For this review, take the finished solid that the model builds, in its own axes (mm). Face numbers are marked on the shaded views. A direction names the side the tool comes from. Coordinates: 2 decimals unless noted, no trailing zeros. Order: outer loops, then holes, each group sorted by start corner. A loop starts at its lowest first (then second) coordinate and runs counter-clockwise, first axis right, second up. Notation, with made-up numbers: M 46.5,20 L 78.5,20 A19 cw 78.5,38 Z; hole C 48.25,38.25 d6. An arc over 180 degrees is marked long. Use CSV: the item, a comma, the result in double quotes.
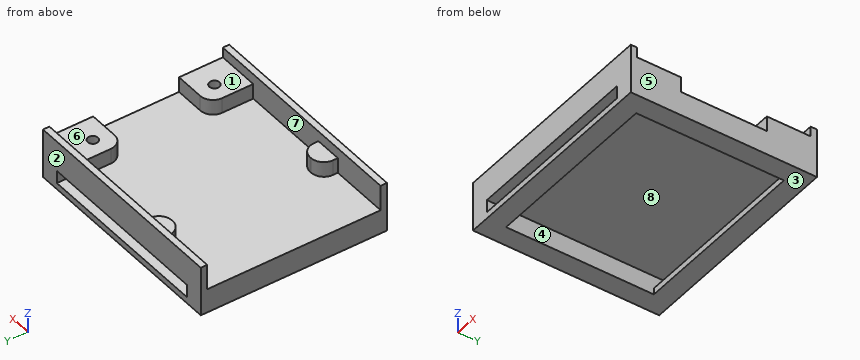
```python
from build123d import *

# Parameters (mm, degrees)
SKETCH2_W               = 29.17
SKETCH2_H               = 34.29
BOSS_EXTRUDE1_DEPTH     = 0.8
SKETCH4_W               = 4.2
SKETCH4_H               = 2.75
SKETCH4_W_2             = 6.61
SKETCH4_H_2             = 6.86
BOSS_EXTRUDE3_DEPTH     = 2.4
SKETCH5_W               = 34.29
SKETCH5_H               = 1
BOSS_EXTRUDE5_DEPTH     = 4
SKETCH6_W               = 3.01
SKETCH6_H               = 29.17
BOSS_EXTRUDE6_DEPTH     = 2
CUT_EXTRUDE1_DEPTH      = 24.10223474
CUT_EXTRUDE1_DEPTH_BACK = 24.10223474
SKETCH8_R               = 0.8
SKETCH9_W               = 34.29
SKETCH9_H               = 29.17
SKETCH9_W_2             = 28.27
SKETCH9_H_2             = 23.15
BOSS_EXTRUDE8_DEPTH     = 1
FILLET1_R               = 2


with BuildPart() as part:
    # Sketch2 → Boss-Extrude1 (new body)
    with BuildSketch(Plane(origin=(0, 0, 0), x_dir=(0, 1, 0), z_dir=(0, 0, 1))):
        Rectangle(SKETCH2_W, SKETCH2_H)
    extrude(amount=BOSS_EXTRUDE1_DEPTH)

    # Sketch4 → Boss-Extrude3 (add)
    with BuildSketch(Plane.XY.offset(0.8)):
        with Locations((-5.745, -12.21)):
            Rectangle(SKETCH4_W, SKETCH4_H)
        with Locations((13.84, -10.155)):
            Rectangle(SKETCH4_W_2, SKETCH4_H_2)
        with Locations((13.84, 10.155)):
            Rectangle(SKETCH4_W_2, SKETCH4_H_2)
        with Locations((-5.745, 12.21)):
            Rectangle(SKETCH4_W, SKETCH4_H)
    extrude(amount=BOSS_EXTRUDE3_DEPTH)

    # Sketch5 → Boss-Extrude5 (add)
    with BuildSketch(Plane.XY.offset(0.8)):
        with Locations((0, 14.085)):
            Rectangle(SKETCH5_W, SKETCH5_H)
        with Locations((0, -14.085)):
            Rectangle(SKETCH5_W, SKETCH5_H)
    extrude(amount=BOSS_EXTRUDE5_DEPTH)

    # Sketch6 → Boss-Extrude6 (add)
    with BuildSketch(Plane(origin=(0, 0, 0), x_dir=(1, 0, 0), z_dir=(0, 0, -1))):
        with Locations((15.64, 0)):
            Rectangle(SKETCH6_W, SKETCH6_H)
        with Locations((-15.64, 0)):
            Rectangle(SKETCH6_W, SKETCH6_H)
    extrude(amount=BOSS_EXTRUDE6_DEPTH)

    # Sketch8 → Cut-Extrude1 (cut, two sides: drawn at the far end of the back side and taken through both)
    with BuildSketch(Plane.XY.offset(3.2).offset(-CUT_EXTRUDE1_DEPTH_BACK)):
        with Locations((13.335, 9.525)):
            Circle(SKETCH8_R)
        with Locations((13.335, -9.525)):
            Circle(SKETCH8_R)
    extrude(amount=CUT_EXTRUDE1_DEPTH + CUT_EXTRUDE1_DEPTH_BACK, mode=Mode.SUBTRACT)

    # Sketch9 → Boss-Extrude8 (add)
    with BuildSketch(Plane(origin=(0, 0, -2), x_dir=(1, 0, 0), z_dir=(0, 0, -1))):
        Rectangle(SKETCH9_W, SKETCH9_H)
        Rectangle(SKETCH9_W_2, SKETCH9_H_2, mode=Mode.SUBTRACT)
    extrude(amount=BOSS_EXTRUDE8_DEPTH)

    # Fillet1
    fillet1_edges = [part.edges().sort_by_distance(p)[0] for p in [
        (-7.845, 10.835, 2),
        (-3.645, 10.835, 2),
        (10.535, 6.725, 2),
        (10.535, -6.725, 2),
        (-3.645, -10.835, 2),
        (-7.845, -10.835, 2),
    ]]
    fillet(fillet1_edges, radius=FILLET1_R)


solid = part.part
```
Item 1: Add section B-B on z = 1.5. State the section outline as (x, y) points (3 decimals).
Solutions:
outline,"M -17.145,-14.585 L 17.145,-14.585 L 17.145,-6.725 L 12.535,-6.725 A2 ccw 10.535,-8.725 L 10.535,-13.585 L -3.645,-13.585 L -3.645,-12.835 A2 ccw -5.645,-10.835 L -5.845,-10.835 A2 ccw -7.845,-12.835 L -7.845,-13.585 L -17.145,-13.585 Z; M -17.145,13.585 L -7.845,13.585 L -7.845,12.835 A2 ccw -5.845,10.835 L -5.645,10.835 A2 ccw -3.645,12.835 L -3.645,13.585 L 10.535,13.585 L 10.535,8.725 A2 ccw 12.535,6.725 L 17.145,6.725 L 17.145,14.585 L -17.145,14.585 Z; hole C 13.335,-9.525 d1.6; hole C 13.335,9.525 d1.6"
Item 2: Add section D-D on y = 5.75. State the section outline as (x, z) points (3 decimals), and give its area (3 significant figures).
Solutions:
outline,"M -17.145,-3 L -14.135,-3 L -14.135,0 L 14.135,0 L 14.135,-3 L 17.145,-3 L 17.145,0.8 L -17.145,0.8 Z"
area,"45.5 mm^2"
Item 3: Clearance check with flat-ended pins moving along their axes: pin 1 Ø0.8 at (y, z) = (-13, 2.5) entering from -X (3 decimals); pin 2 Ø3 at (x, y) = (-5.5, -12) entering from +Z; pin 3 Ø12 at (x, y) = (-1, 4) entering from +Z. State where each tip first meets the part, or that it passes through.
Solutions:
pin 1,"x = -7.845"
pin 2,"z = 3.2"
pin 3,"z = 0.8"
Item 4: Add section A-A on x = 9.5. State the section outline as (y, z) points (3 decimals), and give its area (3 significant figures).
Solutions:
outline,"M -14.585,-3 L -11.575,-3 L -11.575,-2 L -14.585,-2 Z; M -14.585,0 L 14.585,0 L 14.585,4.8 L 13.585,4.8 L 13.585,0.8 L -13.585,0.8 L -13.585,4.8 L -14.585,4.8 Z; M 11.575,-3 L 14.585,-3 L 14.585,-2 L 11.575,-2 Z"
area,"37.4 mm^2"
Item 5: For the marked faces 4, 5, 6, 7 and 8, list the 3-axis set-ups (+Z, -Z, +X, -X, +Y, -Y) from which the entire face can be reached by the end or side of a thin tool; tool diameter is ignored.
Solutions:
face 4,"none"
face 5,"+Z, -Z, +X, +Y, -Y"
face 6,"+Z, +X, -X"
face 7,"+Z"
face 8,"+Y, -Y"
Item 6: Add section C-C on z = -1.5. State the section outline as (x, y) points (3 decimals).
Solutions:
outline,"M -17.145,-14.585 L -14.135,-14.585 L -14.135,14.585 L -17.145,14.585 Z; M 14.135,-14.585 L 17.145,-14.585 L 17.145,14.585 L 14.135,14.585 Z"
Item 7: Draft analysis for pull direction Y (two halves, no side actions). For the marked faces 1, 2 and 3, state which applies: released by +Y, released by -Y, zero draft, split by the parting line, or undercut.
Solutions:
face 1,"undercut"
face 2,"released by +Y"
face 3,"zero draft"
Item 8: To check wall thickness, follow line 1 along Y through (x, z) = (-2.5, 4) (3 decimals); line 2 along X through (y, z) = (9.5, -1.25) (3 decimals); line 3 along X through (y, z) = (-12.75, 2.5) (3 decimals). State the ranges of each line that lie inside material, in increasing order. Write a range as [from, to].
Solutions:
line 1,"[-14.585, -13.585], [13.585, 14.585]"
line 2,"[-17.145, -14.135], [14.135, 17.145]"
line 3,"[-7.843, -3.647], [10.535, 17.145]"
